The model under review builds one solid part; all positions refer to its coordinate system, in mm. Face numbers are marked on the shaded views. A direction names the side the tool comes from. Give positions to 0.01 mm unless a question says otherwise; leave off trailing zeros. Write each loop counter-clockwise with the first axis right and the second up, starting at its lowest first coordinate (ties: lowest second). Pieces come first, ordered by that corner, then holes. Notation, with made-up numbers: (62.25, 22) - (116.25, 22) arc R33 cw to (116.25, 51) - close; hole circle Ø4 at (22.5, 44.5). An arc over 180 degrees is marked (long way). Write item = value, one per line.
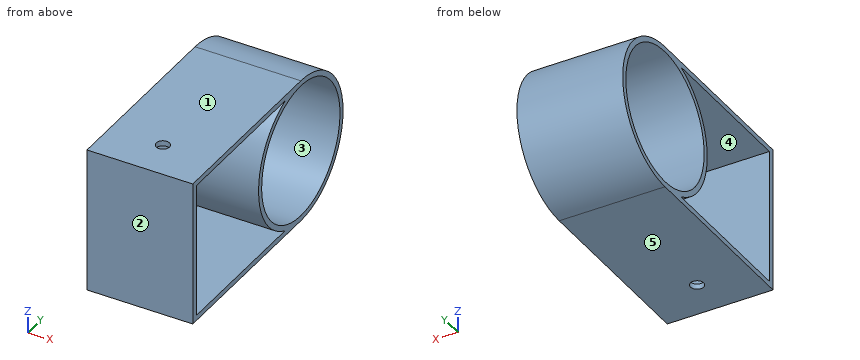
```python
from build123d import *

# Parameters (mm, degrees)
SKETCH1_R           = 25.5
BOSS_EXTRUDE1_DEPTH = 40
SKETCH2_R           = 2.5
CUT_EXTRUDE1_DEPTH  = 98.850406679


with BuildPart() as part:
    # Sketch1 → Boss-Extrude1 (new body)
    with BuildSketch(Plane(origin=(0, 0, 0), x_dir=(0, 0, -1), z_dir=(1, 0, 0))):
        with BuildLine():
            Line((-27.5, 0), (-27.5, -70.354119191))
            Line((-27.5, -70.354119191), (27.5, -70.354119191))
            Line((27.5, -70.354119191), (27.5, 0))
            ThreePointArc((27.5, 0), (0, 27.5), (-27.5, 0))
        make_face()
        Circle(SKETCH1_R, mode=Mode.SUBTRACT)
        with BuildLine():
            Line((-25.5, -10.295630141), (-25.5, -67.945646506))
            Line((-25.5, -67.945646506), (25.5, -67.945646506))
            Line((25.5, -67.945646506), (25.5, -10.295630141))
            ThreePointArc((25.5, -10.295630141), (0, -27.5), (-25.5, -10.295630141))
        make_face(mode=Mode.SUBTRACT)
    extrude(amount=-BOSS_EXTRUDE1_DEPTH)

    # Sketch2 → Cut-Extrude1 (cut, through all)
    with BuildSketch(Plane.XY.offset(27.5)):
        with Locations((-20, -55.354119191)):
            Circle(SKETCH2_R)
    extrude(amount=-CUT_EXTRUDE1_DEPTH, mode=Mode.SUBTRACT)


solid = part.part
```
1. Machinability: for the marked faces 4 and 5, which of the approach directions +Z, -Z, +X, -X, +Y, -Y give a long, thin tool a straight path to every point of the face, cutting with its end or side? Answer none if there is none.
Findings below:
face_4 = +X, -X
face_5 = -Z, +X, -X, +Y, -Y
2. Draft analysis for pull direction Y (two halves, no side actions). For the marked faces 1, 2 and 3, state which applies: +Y half, -Y half, draft (parallel to the pull), parting line (faces both ways), or undercut.
Findings below:
face_1 = draft
face_2 = -Y half
face_3 = undercut
3. Insertion check: P1, Ø3, axis at x = -20, y = -55.35, coming from the -Z side; P2, Ø12, axis at x = -26.5, z = 11, coming from the +Y side; P3, Ø5, axis at x = -15.5, z = 13, coming from the +Y side; P4, Ø3, axis at x = -7.5, z = 14.5, coming from the +Y side. Each pin has a flat end and moves straight along its axis. Give the tip position at first contact, or say it passes through.
Findings below:
P1 = through
P2 = 27.04
P3 = 25.42
P4 = 24.23
4. Take a section at B-B on y = -41.5. Give the boundary of the cut face in (x, z).
Findings below:
outline = (-40, -27.5) - (0, -27.5) - (0, -25.5) - (-40, -25.5) - close; (-40, 25.5) - (0, 25.5) - (0, 27.5) - (-40, 27.5) - close
5. Take a section at C-C on z = 0. Give the boundary of the cut face in (x, y), and give its area (3 significant figures).
Findings below:
outline = (-40, -70.35) - (0, -70.35) - (0, -67.95) - (-40, -67.95) - close; (-40, -27.5) - (0, -27.5) - (0, -25.5) - (-40, -25.5) - close; (-40, 25.5) - (0, 25.5) - (0, 27.5) - (-40, 27.5) - close
area = 256 mm²
6. Take a section at A-A on x = -20. Give the boundary of the cut face in (y, z).
Findings below:
outline = (-70.35, -27.5) - (-57.85, -27.5) - (-57.85, -25.5) - (-67.95, -25.5) - (-67.95, 25.5) - (-57.85, 25.5) - (-57.85, 27.5) - (-70.35, 27.5) - close; (-52.85, -27.5) - (0, -27.5) arc R27.5 ccw to (0, 27.5) - (-52.85, 27.5) - (-52.85, 25.5) - (-10.3, 25.5) arc R27.5 ccw to (-10.3, -25.5) - (-52.85, -25.5) - close; hole circle Ø51 at (0, 0)
7. Take a section at D-D on x = -14. Give the boundary of the cut face in (y, z), and give its area (3 significant figures).
Findings below:
outline = (-70.35, -27.5) - (0, -27.5) arc R27.5 ccw to (0, 27.5) - (-70.35, 27.5) - close; hole (-67.95, -25.5) - (-10.3, -25.5) arc R27.5 cw to (-10.3, 25.5) - (-67.95, 25.5) - close; hole circle Ø51 at (0, 0)
area = 710 mm²
8. For line 1 (Z direction, x = -7.5, y = -49.5); line 2 (Y direction, x = -6, z = 9); line 3 (Z direction, x = -10.5, y = -12), list the stretches that pass through material, from the lowest coordinate up. Write a range as from..to.
Findings below:
line_1 = -27.5..-25.5, 25.5..27.5
line_2 = -70.35..-67.95, -25.99..-23.86, 23.86..25.99
line_3 = -27.5..-25.5, -24.74..-22.5, 22.5..24.74, 25.5..27.5
